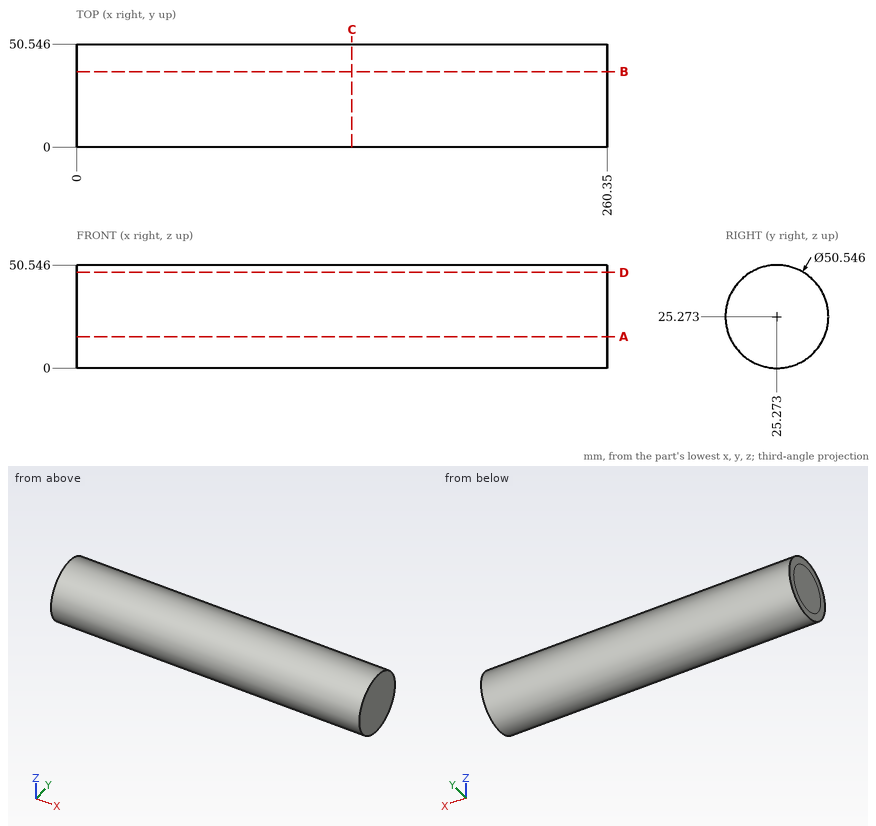
Here's the drawing with two shaded views (mm, measured from the low corner). I have some questions. Give positions to 0.01 mm unless a question says otherwise; leave off trailing zeros. Write each loop counter-clockwise with the first axis right and the second up, starting at its lowest first coordinate (ties: lowest second). Pieces come first, ordered by that corner, then holes. Notation, with made-up numbers: (40, 7.25) - (47, 7.25) arc R15 ccw to (47, 20.25) - close; hole circle Ø11 at (-11, 10). An arc over 180 degrees is marked (long way). One line per item, written item: value. Start each with the question number.
Item 1: Imagine slicing it at A-A, the plane z = 15.5. List the corners of the cut face in (x, y) for me, and give its area (3 significant figures).
Item 2: Please list where these lines run through material, in increasing order: line 1 (Y direction, x = 245, z = 14); line 2 (Y direction, x = 203.5, z = 19.5); line 3 (Z direction, x = 15, y = 23.5). Write a range as from..to.
Item 3: Imagine slicing it at D-D, the plane z = 47. List the corners of the cut face in (x, y) for me, and give its area (3 significant figures).
Item 4: Imagine slicing it at B-B, the plane y = 37. List the corners of the cut face in (x, z) for me, and give its area (3 significant figures).
Item 5: I'm going to push flat-ended pins straight in: pin 1 (1.5 mm diameter, centred on x = 42, y = 8.5, fed in from +Z); pin 2 (5 mm diameter, centred on x = 105, y = 8, fed in from +Z); pin 3 (8 mm diameter, centred on x = 95, y = 37.5, fed in from -Z). Where does each tip first touch, or does it pass through?
Item 6: Imagine slicing it at C-C, the plane x = 135. List the corners of the cut face in (y, z) for me.
Geometry says:
1. outline: (0, 1.97) - (260.35, 1.97) - (260.35, 48.58) - (0, 48.58) - close
1. area: 12,100 mm^2
2. line 1: 2.65..47.89
2. line 2: 0.67..49.88
2. line 3: 0.06..50.48
3. outline: (0, 12.36) - (260.35, 12.36) - (260.35, 38.18) - (0, 38.18) - close
3. area: 6,720 mm^2
4. outline: (0, 2.89) - (260.35, 2.89) - (260.35, 47.66) - (0, 47.66) - close
4. area: 11,700 mm^2
5. pin 1: z = 44.82
5. pin 2: z = 45.78
5. pin 3: z = 1.38
6. outline: circle Ø50.55 at (25.27, 25.27)
